from build123d import *

# Parameters (mm, degrees)
SKETCH1_W           = 20
SKETCH1_H           = 34
BOSS_EXTRUDE1_DEPTH = 4
BOSS_EXTRUDE2_DEPTH = 20
FILLET1_R           = 5
SKETCH3_R           = 1.6
CUT_EXTRUDE1_DEPTH  = 21
SKETCH4_R           = 2.1
CUT_EXTRUDE2_DEPTH  = 5
FILLET2_R           = 2
SKETCH5_W           = 5
SKETCH5_H           = 12
CUT_EXTRUDE3_DEPTH  = 8.872457626


with BuildPart() as part:
    # Sketch1 → Boss-Extrude1 (new body)
    with BuildSketch(Plane.XY):
        with Locations((-10, 17)):
            Rectangle(SKETCH1_W, SKETCH1_H)
    extrude(amount=BOSS_EXTRUDE1_DEPTH)

    # Sketch2 → Boss-Extrude2 (add)
    with BuildSketch(Plane(origin=(0, 0, 0), x_dir=(0, 0, -1), z_dir=(1, 0, 0))):
        with BuildLine():
            Line((-4, 29), (-4, 34))
            Line((-4, 34), (0, 34))
            ThreePointArc((0, 34), (-6.995932864, 35.496746291), (-4, 29))
        make_face()
    extrude(amount=-BOSS_EXTRUDE2_DEPTH)

    # Fillet1
    fillet1_edges = [part.edges().sort_by_distance(p)[0] for p in [
        (-10, 29, 4),
    ]]
    fillet(fillet1_edges, radius=FILLET1_R)

    # Sketch3 → Cut-Extrude1 (cut, through all)
    with BuildSketch(Plane(origin=(0, 0, 0), x_dir=(0, 0, -1), z_dir=(1, 0, 0))):
        with Locations((-3.872457626, 32.997966101)):
            Circle(SKETCH3_R)
    extrude(amount=-CUT_EXTRUDE1_DEPTH, mode=Mode.SUBTRACT)

    # Sketch4 → Cut-Extrude2 (cut, through all)
    with BuildSketch(Plane.XY.offset(4)):
        with Locations((-10, 8)):
            Circle(SKETCH4_R)
    extrude(amount=-CUT_EXTRUDE2_DEPTH, mode=Mode.SUBTRACT)

    # Fillet2
    fillet2_edges = [part.edges().sort_by_distance(p)[0] for p in [
        (0, 0, 2),
        (-20, 0, 2),
    ]]
    fillet(fillet2_edges, radius=FILLET2_R)

    # Sketch5 → Cut-Extrude3 (cut, through all)
    with BuildSketch(Plane(origin=(0, 0, 0), x_dir=(-1, 0, 0), z_dir=(0, 0, -1))):
        with Locations((2.5, 34)):
            Rectangle(SKETCH5_W, SKETCH5_H)
        with Locations((12.5, 34)):
            Rectangle(SKETCH5_W, SKETCH5_H)
    extrude(amount=-CUT_EXTRUDE3_DEPTH, mode=Mode.SUBTRACT)


solid = part.part
Source: CAD feature listing. Evaluate the final solid. Frame: model axes, mm. A direction names the side the tool comes from. Give positions to 0.01 mm unless a question says otherwise; leave off trailing zeros. Write each loop counter-clockwise with the first axis right and the second up, starting at its lowest first coordinate (ties: lowest second). Pieces come first, ordered by that corner, then holes. Notation, with made-up numbers: M 81,-31.5 L 116,-31.5 A20 cw 116,5.5 Z; hole C 33,42 d9. An arc over 180 degrees is marked long. Return JSON: item names as keys, results as strings. Group by question number.
1) Cut plane D-D, the plane y = 12. Output: boundary loops of the cut face in (x, z).
2) Cut plane B-B, the plane x = -11.5. Output: boundary loops of the cut face in (y, z).
3) Set-up query: faces 1 (the face through (-5, 31, 3)), 2 (the face through (-10, 13, 4)), 3 (the face through (-15, 31, 3)), 4 (the face through (0, 15, 2)). Return all of +Z, -Z, +X, -X, +Y, -Y with unobstructed straight access to the full face (end or side cutting, diameter ignored); none if empty.
4) Cut plane C-C, the plane x = -3. Output: boundary loops of the cut face in (y, z).
5) Material intervals for line 1 along X through (y, z) = (35, 1.5); line 2 along Y through (x, z) = (-14.5, 1.5); line 3 along Z through (x, y) = (-12.25, 18), sorted ascending. Write a range as [from, to].
6) Pull-direction query (Y, two-part tool) for faces 5 (the face through (-11.548, 9.419, 2.028)), 6 (the face through (-10, 31, 3)), 7 (the face through (-2, 28, 2)); classes: pulls with the +Y half, pulls with the -Y half, needs draft (parallel to the pull), parting line crosses it, or undercut.
7) Pin query (flat end, axial travel): P1, Ø1.5, axis at y = 28.5, z = 3.5, coming from the +X side; P2, Ø10, axis at x = -4.5, y = 24.5, coming from the +Z side; P3, Ø2.5, axis at y = 31.5, z = 5.5, coming from the +X side; P4, Ø3.5, axis at x = -13, z = 1.5, coming from the +Y side. Return the tip coordinate at first contact, or that it passes through.
8) Cut plane A-A, the plane y = 8. Output: boundary loops of the cut face in (x, z).
Recorded:
{
 "1": {"outline": "M -20,0 L 0,0 L 0,4 L -20,4 Z"},
 "2": {"outline": "M 0,0 L 6.53,0 L 6.53,4 L 0,4 Z; M 9.47,0 L 28,0 L 28,4.61 A5 cw 25.6,4 L 9.47,4 Z"},
 "3": {"face 1": "+Z, -Z, +X, +Y", "face 2": "+Z, +X, -X, -Y", "face 3": "+Z, -Z, +Y", "face 4": "+Z, -Z, +X, +Y, -Y"},
 "4": {"outline": "M 0,0 L 28,0 L 28,4.61 A5 cw 25.6,4 L 0,4 Z"},
 "5": {"line 1": "x = [-20, -15], [-10, -5]", "line 2": "y = [0, 28]", "line 3": "z = [0, 4]"},
 "6": {"face 5": "undercut", "face 6": "needs draft", "face 7": "pulls with the +Y half"},
 "7": {"P1": "stops at x = 0", "P2": "stops at z = 5.84", "P3": "stops at x = -5", "P4": "stops at y = 28"},
 "8": {"outline": "M -20,0 L -12.1,0 L -12.1,4 L -20,4 Z; M -7.9,0 L 0,0 L 0,4 L -7.9,4 Z"}
}
